Input: part model. Units: mm. Frame: model coordinates. Face numbers are marked on the shaded views. A direction names the side the tool comes from. Give positions to 0.01 mm unless a question says otherwise; leave off trailing zeros. Write each loop counter-clockwise with the first axis right and the second up, starting at its lowest first coordinate (ties: lowest second). Pieces come first, ordered by that corner, then holes. Notation, with made-up numbers: (52.5, 41) - (95.5, 41) arc R11 ccw to (95.5, 60) - close; hole circle Ø9 at (88.5, 43). An arc over 180 degrees is marked (long way). Use a Markdown table: item, result. Add a question column.
1. Section query A-A, the plane x = 0. Return loops of the section in (y, z) (1 decimal), plus the area to 3 significant figures.
2. Mould query, pull axis Z, two halves, no side actions, for the marked faces 4, 5 and 6. Classes: released by +Z, released by -Z, zero draft, split by the parting line, or undercut.
3. Section query C-C, the plane z = 0. Return loops of the section in (x, y) (3 decimals).
4. Material intervals for probe 1 along X at (y, z) = (3, 0); probe 2 along Z at (x, y) = (-0.5, 21.5); probe 3 along Y at (x, z) = (5, -12.5), sorted ascending.
5. Set-up query: the marked faces 1, 2 and 3. Return all of +Z, -Z, +X, -X, +Y, -Y with unobstructed straight access to the full face (end or side cutting, diameter ignored); none if empty.
6. Section query B-B, the plane z = -10.5. Return loops of the section in (x, y).
7. Section query D-D, the plane y = 16.25. Return loops of the section in (x, z), plus the area to 3 significant figures.
8. Pin query (flat end, axial travel): pin 1 (3 mm diameter, centred on y = 26.5, z = -13, fed in from -X); pin 2 (12 mm diameter, centred on x = -4.5, z = -15.5, fed in from +Y); pin 3 (1.2 mm diameter, centred on y = 26, z = -11.5, fed in from +X). Return the tip coordinate at first contact, or that it passes through.
```python
from build123d import *

# Parameters (mm, degrees)
SKETCH1_R               = 4.7625
SKETCH1_R_2             = 2.9718
BOSS_EXTRUDE1_DEPTH     = 6.35
SKETCH2_R               = 12.7
SKETCH2_R_2             = 2.9718
BOSS_EXTRUDE3_DEPTH     = 3.175
SKETCH3_R               = 12.7
BOSS_EXTRUDE4_DEPTH     = 19.05
CUT_EXTRUDE1_DEPTH      = 29.575
CUT_EXTRUDE1_DEPTH_BACK = 29.575
SKETCH4_R               = 1.143
SKETCH5_W               = 25.4
SKETCH5_H               = 28.575
CUT_EXTRUDE2_DEPTH      = 38.855587712
BOSS_EXTRUDE6_START     = 6.35
BOSS_EXTRUDE6_DEPTH     = 6.35
SKETCH8_W               = 18.623587624
SKETCH8_H               = 3.175
BOSS_EXTRUDE7_DEPTH     = 11.1125
SKETCH9_W               = 18.623587624
SKETCH9_H               = 0.79375
BOSS_EXTRUDE8_DEPTH     = 9.525


with BuildPart() as part:
    # Sketch1 → Boss-Extrude1 (new body)
    with BuildSketch(Plane(origin=(0, 0, 0), x_dir=(1, 0, 0), z_dir=(0, 1, 0))):
        with Locations(Location((0, 0, 0), (0, 0, 270))):
            Circle(SKETCH1_R)
        with Locations(Location((0, 0, 0), (0, 0, 270))):
            Circle(SKETCH1_R_2, mode=Mode.SUBTRACT)
    extrude(amount=BOSS_EXTRUDE1_DEPTH)

    # Sketch2 → Boss-Extrude3 (add)
    with BuildSketch(Plane(origin=(0, 6.35, 0), x_dir=(1, 0, 0), z_dir=(0, 1, 0))):
        with Locations(Location((0, 0, 0), (0, 0, 270))):
            Circle(SKETCH2_R)
        with Locations(Location((0, 0, 0), (0, 0, 270))):
            Circle(SKETCH2_R_2, mode=Mode.SUBTRACT)
    extrude(amount=BOSS_EXTRUDE3_DEPTH)

    # Sketch3 → Boss-Extrude4 (add)
    with BuildSketch(Plane(origin=(0, 9.525, 0), x_dir=(1, 0, 0), z_dir=(0, 1, 0))):
        with Locations(Location((0, 0, 0), (0, 0, 270))):
            Circle(SKETCH3_R)
        with BuildLine():
            Line((-4.983839885, 6.096), (4.983839885, 6.096))
            ThreePointArc((4.983839885, 6.096), (7.874, 0), (4.983839885, -6.096))
            Line((4.983839885, -6.096), (-4.983839885, -6.096))
            ThreePointArc((-4.983839885, -6.096), (-7.874, 0), (-4.983839885, 6.096))
        make_face(mode=Mode.SUBTRACT)
    extrude(amount=BOSS_EXTRUDE4_DEPTH)

    # Sketch4 → Cut-Extrude1 (cut, two sides: drawn at the far end of the back side and taken through both)
    with BuildSketch(Plane.XZ.offset(-6.35).offset(-CUT_EXTRUDE1_DEPTH_BACK)):
        with Locations(Location((-4.399409051, -0.635, 0), (0, 0, 269.056983799))):
            Circle(SKETCH4_R)
        with Locations(Location((4.399409051, 0.635, 0), (0, 0, 287.369437604))):
            Circle(SKETCH4_R)
    extrude(amount=CUT_EXTRUDE1_DEPTH + CUT_EXTRUDE1_DEPTH_BACK, mode=Mode.SUBTRACT)

    # Sketch5 → Cut-Extrude2 (cut, through all)
    with BuildSketch(Plane.XY.offset(-8.636)):
        with Locations((0, 14.2875)):
            Rectangle(SKETCH5_W, SKETCH5_H)
    extrude(amount=-CUT_EXTRUDE2_DEPTH, mode=Mode.SUBTRACT)

    # Sketch7 → Boss-Extrude6 (add)
    with BuildSketch(Plane.XZ.offset(-6.35).offset(BOSS_EXTRUDE6_START)):
        with BuildLine():
            Line((-9.311793812, -8.636), (9.311793812, -8.636))
            ThreePointArc((9.311793812, -8.636), (0, 12.7), (-9.311793812, -8.636))
        make_face()
        with BuildLine():
            ThreePointArc((-4.740630835, 0.455878863), (-5.530685664, -0.798285714), (-4.418220539, -1.77784519))
            ThreePointArc((-4.418220539, -1.77784519), (0.680357143, -4.713652555), (4.740630835, -0.455878863))
            ThreePointArc((4.740630835, -0.455878863), (5.530685664, 0.798285714), (4.418220539, 1.77784519))
            ThreePointArc((4.418220539, 1.77784519), (-0.680357143, 4.713652555), (-4.740630835, 0.455878863))
        make_face(mode=Mode.SUBTRACT)
    extrude(amount=-BOSS_EXTRUDE6_DEPTH)

    # Sketch8 → Boss-Extrude7 (add)
    with BuildSketch(Plane(origin=(0, 0, -8.636), x_dir=(-1, 0, 0), z_dir=(0, 0, -1))):
        with Locations((0, 1.5875)):
            Rectangle(SKETCH8_W, SKETCH8_H)
        with Locations((0, 25.7683)):
            Rectangle(SKETCH8_W, SKETCH8_H)
    extrude(amount=BOSS_EXTRUDE7_DEPTH)

    # Sketch9 → Boss-Extrude8 (add)
    with BuildSketch(Plane(origin=(0, 0, -8.636), x_dir=(-1, 0, 0), z_dir=(0, 0, -1))):
        with Locations((0, 3.571875)):
            Rectangle(SKETCH9_W, SKETCH9_H)
        with Locations((0, 23.783925)):
            Rectangle(SKETCH9_W, SKETCH9_H)
    extrude(amount=BOSS_EXTRUDE8_DEPTH)


solid = part.part
```
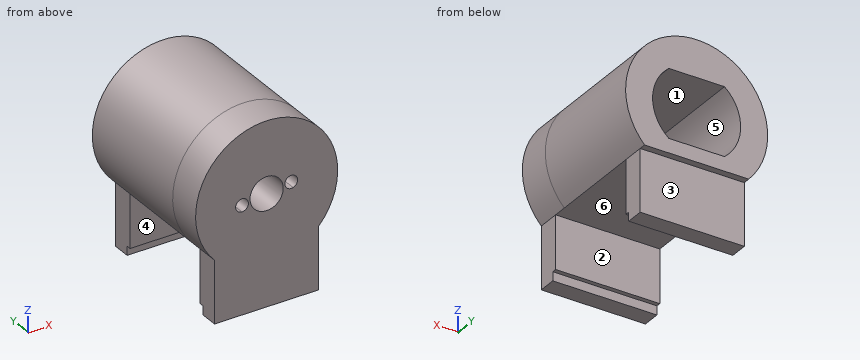
Result sheet:
| question | item | result |
|---|---|---|
| 1 | outline | (0, -19.7) - (3.2, -19.7) - (3.2, -18.2) - (4, -18.2) - (4, -8.6) - (23.4, -8.6) - (23.4, -18.2) - (24.2, -18.2) - (24.2, -19.7) - (27.4, -19.7) - (27.4, -8.6) - (28.6, -8.6) - (28.6, -6.1) - (9.5, -6.1) - (9.5, -3) - (0, -3) - close; (0, 3) - (9.5, 3) - (9.5, 6.1) - (28.6, 6.1) - (28.6, 12.7) - (0, 12.7) - close |
| 1 | area | 406 mm² |
| 2 | face 4 | zero draft |
| 2 | face 5 | undercut |
| 2 | face 6 | released by -Z |
| 3 | outline | (-12.7, 0) - (-5.35, 0) - (-5.35, 9.525) - (-7.874, 9.525) - (-7.874, 28.575) - (-12.7, 28.575) - close; (-3.449, 0) - (-2.972, 0) - (-2.972, 9.525) - (-3.449, 9.525) - close; (2.972, 0) - (3.449, 0) - (3.449, 9.525) - (2.972, 9.525) - close; (5.35, 0) - (12.7, 0) - (12.7, 28.575) - (7.874, 28.575) - (7.874, 9.525) - (5.35, 9.525) - close |
| 4 | probe 1 | x = -12.7 to -5.35, -3.45 to -2.97, 2.97 to 3.45, 5.35 to 12.7 |
| 4 | probe 2 | z = -8.64 to -6.1, 6.1 to 12.69 |
| 4 | probe 3 | y = 0 to 3.97, 23.39 to 27.36 |
| 5 | face 1 | +Y |
| 5 | face 2 | -Z, +X, -X |
| 5 | face 3 | -Z, +X, -X, +Y |
| 6 | outline | (-9.31, 0) - (9.31, 0) - (9.31, 3.97) - (-9.31, 3.97) - close; (-9.31, 23.39) - (9.31, 23.39) - (9.31, 27.36) - (-9.31, 27.36) - close |
| 7 | outline | (-9.31, -8.64) - (9.31, -8.64) arc R12.7 ccw (long way) to start; hole (-4.98, -6.1) - (4.98, -6.1) arc R7.87 ccw to (4.98, 6.1) - (-4.98, 6.1) arc R7.87 ccw to start |
| 7 | area | 284 mm² |
| 8 | pin 1 | stops at x = -9.31 |
| 8 | pin 2 | stops at y = 27.36 |
| 8 | pin 3 | stops at x = 9.31 |
